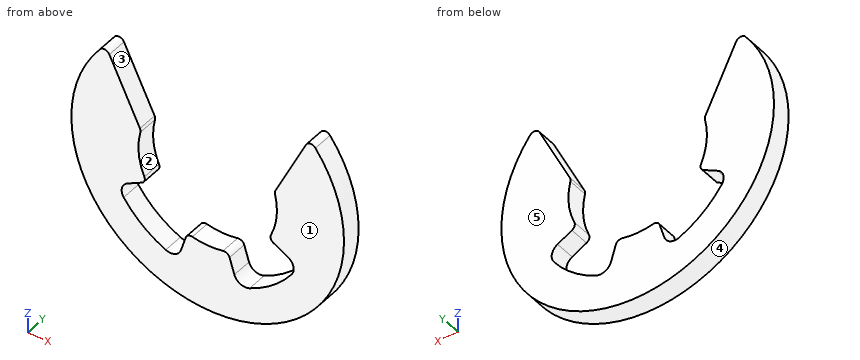
from build123d import *

# Parameters (mm, degrees)
BOSS_EXTRUDE2_DEPTH = 0.9


with BuildPart() as part:
    # Sketch2 → Boss-Extrude2 (new body)
    with BuildSketch(Plane(origin=(0, 0, 0), x_dir=(1, 0, 0), z_dir=(0, 1, 0))):
        with BuildLine():
            Line((-0.980410681, 3.193555213), (-1.194279845, 3.890205091))
            ThreePointArc((-1.194279845, 3.890205091), (-1.465461571, 4.198694788), (-1.876197196, 4.1999862))
            ThreePointArc((-1.876197196, 4.1999862), (-2.921430522, 3.553201895), (-3.758071134, 2.652715844))
            ThreePointArc((-3.758071134, 2.652715844), (-3.836204314, 2.249478162), (-3.585956323, 1.92377682))
            Line((-3.585956323, 1.92377682), (-2.943790684, 1.579270847))
            ThreePointArc((-2.943790684, 1.579270847), (-2.825493737, 1.440063272), (-2.833470582, 1.257554952))
            ThreePointArc((-2.833470582, 1.257554952), (-3.087628894, 0.276672749), (-3.011906881, -0.733768997))
            ThreePointArc((-3.011906881, -0.733768997), (-3.006278091, -0.820065307), (-3.030387689, -0.903116277))
            Line((-3.030387689, -0.903116277), (-4.400044699, -3.693030626))
            ThreePointArc((-4.400044699, -3.693030626), (-4.599153629, -3.831574182), (-4.822086086, -3.735971866))
            ThreePointArc((-4.822086086, -3.735971866), (0, 6.1), (4.822086086, -3.735971866))
            ThreePointArc((4.822086086, -3.735971866), (4.599153629, -3.831574182), (4.400044699, -3.693030626))
            Line((4.400044699, -3.693030626), (3.030387689, -0.903116277))
            ThreePointArc((3.030387689, -0.903116277), (3.006278091, -0.820065307), (3.011906881, -0.733768997))
            ThreePointArc((3.011906881, -0.733768997), (3.087628894, 0.276672749), (2.833470582, 1.257554952))
            ThreePointArc((2.833470582, 1.257554952), (2.825493737, 1.440063272), (2.943790684, 1.579270847))
            Line((2.943790684, 1.579270847), (3.585956323, 1.92377682))
            ThreePointArc((3.585956323, 1.92377682), (3.836204314, 2.249478162), (3.758071134, 2.652715844))
            ThreePointArc((3.758071134, 2.652715844), (2.921430522, 3.553201895), (1.876197196, 4.1999862))
            ThreePointArc((1.876197196, 4.1999862), (1.465461571, 4.198694788), (1.194279845, 3.890205091))
            Line((1.194279845, 3.890205091), (0.980410681, 3.193555213))
            ThreePointArc((0.980410681, 3.193555213), (0.866697189, 3.050579136), (0.68608945, 3.023124421))
            ThreePointArc((0.68608945, 3.023124421), (0, 3.1), (-0.68608945, 3.023124421))
            ThreePointArc((-0.68608945, 3.023124421), (-0.866697189, 3.050579136), (-0.980410681, 3.193555213))
        make_face()
    extrude(amount=BOSS_EXTRUDE2_DEPTH)


solid = part.part
For this review, take the finished solid that the model builds, in its own axes (mm). Face numbers are marked on the shaded views. A direction names the side the tool comes from. Coordinates: 2 decimals unless noted, no trailing zeros. Order: outer loops, then holes, each group sorted by start corner. A loop starts at its lowest first (then second) coordinate and runs counter-clockwise, first axis right, second up. Notation, with made-up numbers: (60, -29.5) -> (117, -29.5) arc R24 cw to (117, -6.5) -> close; hole circle Ø9 at (9, 80). An arc over 180 degrees is marked (long way). Return JSON: item names as keys, results as strings.
1. We need section D-D on x = 0. Write out the cut boundary in (y, z), and give its area (3 significant figures).
Answer block:
{"outline": "(0, -6.1) -> (0.9, -6.1) -> (0.9, -3.1) -> (0, -3.1) -> close", "area": "2.70 mm²"}
2. We need section B-B on y = 0.65. Write out the cut boundary in (x, z).
Answer block:
{"outline": "(-4.82, 3.74) arc R6.1 ccw (long way) to (4.82, 3.74) arc R0.25 ccw to (4.4, 3.69) -> (3.03, 0.9) arc R0.25 ccw to (3.01, 0.73) arc R3.1 cw to (2.83, -1.26) arc R0.25 ccw to (2.94, -1.58) -> (3.59, -1.92) arc R0.5 cw to (3.76, -2.65) arc R4.6 cw to (1.88, -4.2) arc R0.5 cw to (1.19, -3.89) -> (0.98, -3.19) arc R0.25 ccw to (0.69, -3.02) arc R3.1 cw to (-0.69, -3.02) arc R0.25 ccw to (-0.98, -3.19) -> (-1.19, -3.89) arc R0.5 cw to (-1.88, -4.2) arc R4.6 cw to (-3.76, -2.65) arc R0.5 cw to (-3.59, -1.92) -> (-2.94, -1.58) arc R0.25 ccw to (-2.83, -1.26) arc R3.1 cw to (-3.01, 0.73) arc R0.25 ccw to (-3.03, 0.9) -> (-4.4, 3.69) arc R0.25 ccw to start"}
3. For line 1 (X direction, y = 0.2, z = -3.75); line 2 (X direction, y = 0.4, z = -3.25); line 3 (Z direction, x = 3.25, y = 0.4), list the stretches that pass through material, from the lowest coordinate up. Write a range as from..to.
Answer block:
{"line 1": "-4.81..-2.66, -1.15..1.15, 2.66..4.81", "line 2": "-5.16..-3.26, -1..1, 3.26..5.16", "line 3": "-5.16..-3.26, -1.74..1.35"}
4. Machinability: for the marked faces 1 and 2, which of the approach directions +Z, -Z, +X, -X, +Y, -Y give a long, thin tool a straight path to every point of the face, cutting with its end or side? Answer none if there is none.
Answer block:
{"face 1": "+Z, -Z, +X, -X, -Y", "face 2": "+Y, -Y"}
5. We need section A-A on z = 0. Write out the cut boundary in (x, y).
Answer block:
{"outline": "(-6.1, 0) -> (-3.1, 0) -> (-3.1, 0.9) -> (-6.1, 0.9) -> close; (3.1, 0) -> (6.1, 0) -> (6.1, 0.9) -> (3.1, 0.9) -> close"}
6. For pin 1 Ø1.5 at (x, z) = (-0.5, -0.5) entering from -Y, flat-tipped, find the tip position at first contact; note if it passes through.
Answer block:
{"pin 1": "through"}
7. We need section C-C on z = 1.5. Write out the cut boundary in (x, y), and give its area (3 significant figures).
Answer block:
{"outline": "(-5.91, 0) -> (-3.32, 0) -> (-3.32, 0.9) -> (-5.91, 0.9) -> close; (3.32, 0) -> (5.91, 0) -> (5.91, 0.9) -> (3.32, 0.9) -> close", "area": "4.66 mm²"}
8. The part is to be moulded in two halves that separate along X. For the marked faces 3, 4 and 5, say which applies: +X half, -X half, draft (parallel to the pull), parting line (faces both ways), or undercut.
Answer block:
{"face 3": "undercut", "face 4": "parting line", "face 5": "draft"}
